from build123d import *

# Parameters (mm, degrees)
CUT_EXTRUDE2_DEPTH = 6.604


with BuildPart() as part:
    # Sketch2 → Revolve1 (revolve)
    with BuildSketch(Plane.XY):
        Polygon((60.96, 6.35), (60.96, 0), (54.102, 0), (50.927, 3.175), (41.275, 3.175), (41.275, 6.35), align=None)
    revolve(axis=Axis((60.96, 0, 0), (-1, 0, 0)))

    # Sketch8 → Cut-Extrude2 (cut)
    with BuildSketch(Plane(origin=(60.96, 0, 0), x_dir=(0, 0, -1), z_dir=(1, 0, 0))):
        with BuildLine():
            Line((2.776494522, 2.286), (-2.776494522, 2.286))
            ThreePointArc((-2.776494522, 2.286), (-3.596486873, 0), (-2.776494522, -2.286))
            Line((-2.776494522, -2.286), (2.776494522, -2.286))
            ThreePointArc((2.776494522, -2.286), (3.385287575, -1.214308801), (3.596486873, 0))
            ThreePointArc((3.596486873, 0), (3.385287575, 1.214308801), (2.776494522, 2.286))
        make_face()
    extrude(amount=-CUT_EXTRUDE2_DEPTH, mode=Mode.SUBTRACT)


solid = part.part
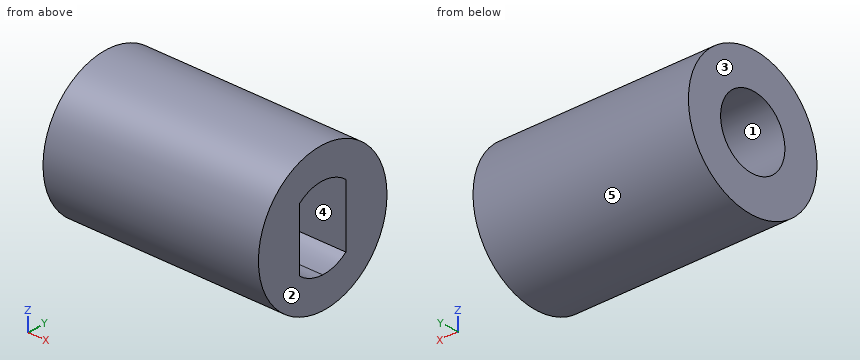
Verification items for the finished model (mm, model axes). Face numbers are marked on the shaded views. A direction names the side the tool comes from. Coordinates: 2 decimals unless noted, no trailing zeros. Order: outer loops, then holes, each group sorted by start corner. A loop starts at its lowest first (then second) coordinate and runs counter-clockwise, first axis right, second up. Notation, with made-up numbers: M 10.5,4 L 49.5,4 A33 ccw 49.5,39 Z; hole C 71,22 d3. An arc over 180 degrees is marked long. Return JSON: item names as keys, results as strings.
1) Release check for a two-part mould opening along Z. For the marked faces 3, 4 and 5 record: +Z half, -Z half, draft (parallel to the pull), parting line (faces both ways), or undercut.
Answer list:
{"face 3": "draft", "face 4": "undercut", "face 5": "parting line"}
2) Cross-section at A-A, the plane x = 58. Record the boundary of the cut face in (y, z), and give its area (3 significant figures).
Answer list:
{"outline": "C 0,0 d12.7; hole M -2.29,-2.78 A3.6 ccw 2.29,-2.78 L 2.29,2.78 A3.6 ccw -2.29,2.78 Z", "area": "96.2 mm2"}
3) Cross-section at C-C, the plane x = 46.25. Record the boundary of the cut face in (y, z) (3 decimals), and give its area (3 significant figures).
Answer list:
{"outline": "C 0,0 d12.7; hole C 0,0 d6.35", "area": "95.0 mm2"}
4) Thickness scan on L1, parallel to Z at x = 43, y = 0 (3 decimals); L2, parallel to Y at x = 58, z = 1.75. Record the ranges inside material, lowest first. Write a range as [from, to].
Answer list:
{"L1": "[-6.35, -3.175], [3.175, 6.35]", "L2": "[-6.1, -2.29], [2.29, 6.1]"}
5) Access from +Z, -Z, +X, -X, +Y, -Y to the whole of each face (thin tool, end or side, straight path). Record for the marked faces 1 and 2.
Answer list:
{"face 1": "-X", "face 2": "+Z, -Z, +X, +Y, -Y"}
6) Cross-section at B-B, the plane y = -5. Record the boundary of the cut face in (x, z) (3 decimals), and give its area (3 significant figures).
Answer list:
{"outline": "M 41.275,-3.914 L 60.96,-3.914 L 60.96,3.914 L 41.275,3.914 Z", "area": "154 mm2"}
7) Gauge pin test, flat ends, axial feed: pin 1 (5 mm diameter, centred on x = 50.5, y = 5, fed in from +Z); pin 2 (1.4 mm diameter, centred on y = 0.5, z = -1, fed in from +X); pin 3 (1.5 mm diameter, centred on x = 44, z = 4, fed in from +Y). Record the tip position at first contact, or that the pin passes through.
Answer list:
{"pin 1": "z = 5.84", "pin 2": "x = 54.36", "pin 3": "y = 5.46"}
8) Cross-section at D-D, the plane x = 52.25. Record the boundary of the cut face in (y, z), and give its area (3 significant figures).
Answer list:
{"outline": "C 0,0 d12.7; hole C 0,0 d3.7", "area": "116 mm2"}
